The model under review builds one solid part; all positions refer to its coordinate system, in mm. A direction names the side the tool comes from. Give positions to 0.01 mm unless a question says otherwise; leave off trailing zeros. Loops run counter-clockwise (first coordinate to the right, second up) from the corner with the lowest first, then second, coordinate; pieces in that order, holes last. Notation, with made-up numbers: M 9,12.5 L 65,12.5 A6 cw 65,16.5 Z; hole C -8,44.5 d4. An arc over 180 degrees is marked long. Put each result on its own line as item: value. Start each with the question number.
from build123d import *

# Parameters (mm, degrees)
F1_DEPTH = 25
F4_DEPTH = 25
F5_DEPTH = 25


with BuildPart() as f1:
    # F0 (on Top) → F1 (new body)
    with BuildSketch(Plane.XY):
        with BuildLine():
            ThreePointArc((0, -25.2255909145), (-9.9045261741, -35.1301170886), (0, -45.0346432626))
            Line((0, -45.0346432626), (39.8768223822, -45.0346432626))
            Line((39.8768223822, -45.0346432626), (49.781344831, -48.7488396466))
            Line((49.781344831, -48.7488396466), (49.781344831, -19.9638102204))
            Line((49.781344831, -19.9638102204), (39.8768223822, -25.2255909145))
            Line((39.8768223822, -25.2255909145), (0, -25.2255909145))
        make_face()
    extrude(amount=F1_DEPTH)

    # F2 (on face) → F4 (join)
    with BuildSketch(Plane.XY.offset(25)):
        with BuildLine():
            Line((39.8768223822, -25.2255909145), (0, -25.2255909145))
            ThreePointArc((0, -25.2255909145), (-9.9045261741, -35.1301170886), (0, -45.0346432626))
            Line((0, -45.0346432626), (39.8768223822, -45.0346432626))
            Line((39.8768223822, -45.0346432626), (49.781344831, -48.7488396466))
            Line((49.781344831, -48.7488396466), (49.781344831, -19.9638102204))
            Line((49.781344831, -19.9638102204), (39.8768223822, -25.2255909145))
        make_face()
    extrude(amount=-F4_DEPTH)

    # F3 (on face) → F5 (cut)
    with BuildSketch(Plane.XY.offset(25)):
        with BuildLine():
            Line((8.6823031306, -32.4443913996), (0, -32.7490344644))
            ThreePointArc((0, -32.7490344644), (-5.4739792074, -36.4047400653), (0, -40.0604456663))
            ThreePointArc((0, -40.0604456663), (2.12452123, -36.2934819265), (6.4182874872, -36.8103741808))
            ThreePointArc((6.4182874872, -36.8103741808), (7.8913776241, -38.1191729594), (8.6357264586, -39.9436985434))
            Line((8.6357264586, -39.9436985434), (18.1262083352, -38.6662621896))
            ThreePointArc((18.1262083352, -38.6662621896), (21.7819157988, -34.7755161234), (25.4376232624, -38.6662621896))
            Line((25.4376232624, -38.6662621896), (37.927955389, -42.4975827336))
            Line((37.927955389, -42.4975827336), (49.781344831, -44.9290481875))
            Line((49.781344831, -44.9290481875), (49.781344831, -26.9712014124))
            Line((49.781344831, -26.9712014124), (35.1861715317, -32.4443913996))
            ThreePointArc((35.1861715317, -32.4443913996), (31.0735022649, -38.6662621896), (26.9608329982, -32.4443913996))
            Line((26.9608329982, -32.4443913996), (19.0401375294, -32.4443913996))
            ThreePointArc((19.0401375294, -32.4443913996), (16.6761777926, -36.8994118679), (11.6438215498, -37.2324338722))
            ThreePointArc((11.6438215498, -37.2324338722), (9.374780297, -35.3259838728), (8.6823031306, -32.4443913996))
        make_face()
        with BuildLine():
            ThreePointArc((8.6357264586, -39.9436985434), (7.8913776241, -38.1191729594), (6.4182874872, -36.8103741808))
            ThreePointArc((6.4182874872, -36.8103741808), (7.4813175027, -38.2742394866), (7.7683748677, -40.0604456663))
            Line((7.7683748677, -40.0604456663), (8.6357264586, -39.9436985434))
        make_face()
        with BuildLine():
            ThreePointArc((18.1262083352, -32.4443913996), (16.2192131955, -36.6447435476), (11.6438215498, -37.2324338722))
            ThreePointArc((11.6438215498, -37.2324338722), (16.6761777926, -36.8994118679), (19.0401375294, -32.4443913996))
            Line((19.0401375294, -32.4443913996), (18.1262083352, -32.4443913996))
        make_face()
    extrude(amount=-F5_DEPTH, mode=Mode.SUBTRACT)


solid = f1.part
(1) We need section B-B, the plane z = 4.75. Write out the cut boundary in (x, y), plus the area to 3 significant figures.
(2) We need section C-C, the plane x = 10. Write out the cut boundary in (y, z), plus the area to 3 significant figures.
(3) For faces 1 (the flat face through (20, -25.226, 12)), 2 (the flat face through (23, -32.444, 13)), 3 (the flat face through (42.59, -29.67, 12.68)), 4 (the flat face through (20, -45.035, 12)), 5 (the flat face through (49.781, -47, 12)), list the 3-axis set-ups (+Z, -Z, +X, -X, +Y, -Y) from which the entire face can be reached by the end or side of a thin tool; tool diameter is ignored.
(4) To check wall thickness, follow L1, parallel to X at y = -33.5, z = 18.25; L2, parallel to X at y = -36.75, z = 10; L3, parallel to X at y = -35.5, z = 17. State the ranges of each line that lie inside material, in increasing order. Write a range as [from, to].
(5) We need section D-D, the plane y = -41.75. Write out the cut boundary in (x, z), plus the area to 3 significant figures.
(6) We need section A-A, the plane x = 41.5. Write out the cut boundary in (y, z).
(7) Draft analysis for pull direction Y (two halves, no side actions). For faces 6 (the flat face through (49.781, -24, 12)), 7 (the flat face through (44.76, -46.866, 12.325)), 8 (the flat face through (31.595, -40.555, 12.675)), 9 (the cylindrical face through (-5.472, -36.296, 12.675)), state which applies: +Y half, -Y half, draft (parallel to the pull), parting line (faces both ways), or undercut.
(8) Insertion check: pin 1 (1 mm diameter, centred on x = 21.5, z = 7.5, fed in from -Y); pin 2 (8 mm diameter, centred on y = -30, z = 12.5, fed in from -X); pin 3 (2 mm diameter, centred on x = 0, z = 8, fed in from +Y); pin 4 (10.5 mm diameter, centred on x = -1.52, y = -36.4, fed in from +Z). Each pin has a flat end and moves straight along its axis. Give the tip position at first contact, or say it passes through.
Check sheet entries:
1. outline: M 0,-45.03 L 39.88,-45.03 L 49.78,-48.75 L 49.78,-44.93 L 37.93,-42.5 L 25.44,-38.67 A3.66 ccw long 18.13,-38.67 L 7.77,-40.06 A3.9 ccw long 0,-40.06 A3.96 cw long 0,-32.75 L 8.68,-32.44 A4.74 ccw long 18.13,-32.44 L 26.96,-32.44 A4.47 ccw long 35.19,-32.44 L 49.78,-26.97 L 49.78,-19.96 L 39.88,-25.23 L 0,-25.23 A9.9 ccw Z
1. area: 833 mm²
2. outline: M -45.03,0 L -39.76,0 L -39.76,25 L -45.03,25 Z; M -36.13,0 L -25.23,0 L -25.23,25 L -36.13,25 Z
2. area: 404 mm²
3. face 1: +Z, -Z, -X, +Y
3. face 2: +Z, -Z
3. face 3: +Z, -Z, +X
3. face 4: +Z, -Z, -X, -Y
3. face 5: +Z, -Z, +X, +Y, -Y
4. L1: x = [-9.77, -4.2], [8.71, 18.1], [26.66, 35.49]
4. L2: x = [-9.77, -5.46], [1.42, 6.35], [10.74, 16.07], [18.53, 25.03], [27.4, 34.74]
4. L3: x = [-9.9, -5.37], [9.49, 17.32], [19.6, 23.97], [26.8, 35.35]
5. outline: M -7.37,0 L 35.49,0 L 35.49,25 L -7.37,25 Z
5. area: 1,070 mm²
6. outline: M -45.64,0 L -43.23,0 L -43.23,25 L -45.64,25 Z; M -30.08,0 L -24.36,0 L -24.36,25 L -30.08,25 Z
7. face 6: draft
7. face 7: -Y half
7. face 8: undercut
7. face 9: undercut
8. pin 1: stops at y = -45.03
8. pin 2: stops at x = -9.84
8. pin 3: stops at y = -25.23
8. pin 4: stops at z = 25
